```python
from build123d import *

# Parameters (mm, degrees)
SKETCH1_W           = 42
SKETCH1_H           = 42
SKETCH1_W_2         = 40
SKETCH1_H_2         = 40
BOSS_EXTRUDE1_DEPTH = 10
SKETCH3_W           = 2
SKETCH3_H           = 40
BOSS_EXTRUDE2_DEPTH = 40
SKETCH5_W           = 40
SKETCH5_H           = 1
CUT_EXTRUDE1_DEPTH  = 10
SKETCH6_W           = 40
SKETCH6_H           = 1
CUT_EXTRUDE2_DEPTH  = 10


with BuildPart() as part:
    # Sketch1 → Boss-Extrude1 (new body)
    with BuildSketch(Plane.XY):
        Rectangle(SKETCH1_W, SKETCH1_H)
        Rectangle(SKETCH1_W_2, SKETCH1_H_2, mode=Mode.SUBTRACT)
    extrude(amount=BOSS_EXTRUDE1_DEPTH)

    # Sketch3 → Boss-Extrude2 (add)
    with BuildSketch(Plane(origin=(-20, 0, 0), x_dir=(0, 0, -1), z_dir=(1, 0, 0))):
        with Locations((-1, 0)):
            Rectangle(SKETCH3_W, SKETCH3_H)
    extrude(amount=BOSS_EXTRUDE2_DEPTH)

    # Sketch5 → Cut-Extrude1 (cut)
    with BuildSketch(Plane.XY.offset(10)):
        with Locations((0, 20.5)):
            Rectangle(SKETCH5_W, SKETCH5_H)
    extrude(amount=-CUT_EXTRUDE1_DEPTH, mode=Mode.SUBTRACT)

    # Sketch6 → Cut-Extrude2 (cut)
    with BuildSketch(Plane.XY.offset(10)):
        with Locations((0, -20.5)):
            Rectangle(SKETCH6_W, SKETCH6_H)
    extrude(amount=-CUT_EXTRUDE2_DEPTH, mode=Mode.SUBTRACT)


solid = part.part
```
The model under review builds one solid part; all positions refer to its coordinate system, in mm. A direction names the side the tool comes from. Give positions to 0.01 mm unless a question says otherwise; leave off trailing zeros. Write each loop counter-clockwise with the first axis right and the second up, starting at its lowest first coordinate (ties: lowest second). Pieces come first, ordered by that corner, then holes. Notation, with made-up numbers: (-9, 58) - (8, 58) arc R23 cw to (8, 71) - close; hole circle Ø5 at (50, 76). An arc over 180 degrees is marked (long way). Answer in a Markdown table with one row per item. Add a question column.
1. Insertion check: P1, Ø3, axis at x = -14, y = 11, coming from the +Z side; P2, Ø1, axis at x = 7, z = 1, coming from the -Y side; P3, Ø2, axis at x = 6.5, z = 0.5, coming from the +Y side. Each pin has a flat end and moves straight along its axis. Give the tip position at first contact, or say it passes through.
2. We need section B-B on y = 12. Write out the cut boundary in (x, z), then the cut area to 3 significant figures.
3. Draft analysis for pull direction X (two halves, no side actions). For faces 4 (the flat face through (20.5, 21, 4.9)), 5 (the flat face through (-21, 0, 5)), 6 (the flat face through (0, -20, 1)), state which applies: +X half, -X half, draft (parallel to the pull), parting line (faces both ways), or undercut.
4. Tool access review of faces 1 (the flat face through (20.5, 0.3, 10)), 2 (the flat face through (0, 20, 1)), 3 (the flat face through (0, 0, 2)): name each direction out of +Z, -Z, +X, -X, +Y, -Y from which nothing blocks a thin tool from reaching the whole face with its end or side.
5. We need section A-A on z = 3. Write out the cut boundary in (x, y).
6. Wall thickness on line 1 along X through (y, z) = (-17, 2.75); line 2 along Z through (x, y) = (17.5, -16.5): over which ranges is each line inside the solid? List them lowest first. Write a range as [from, to].
7. We need section C-C on x = 6. Write out the cut boundary in (y, z), then the cut area to 3 significant figures.
Ans:
| question | item | result |
|---|---|---|
| 1 | P1 | stops at z = 2 |
| 1 | P2 | stops at y = -20 |
| 1 | P3 | stops at y = 20 |
| 2 | outline | (-21, 0) - (21, 0) - (21, 10) - (20, 10) - (20, 2) - (-20, 2) - (-20, 10) - (-21, 10) - close |
| 2 | area | 100 mm^2 |
| 3 | face 4 | draft |
| 3 | face 5 | -X half |
| 3 | face 6 | undercut |
| 4 | face 1 | +Z, +X, -X, +Y, -Y |
| 4 | face 2 | +Z, -Z, +Y |
| 4 | face 3 | +Z, +Y, -Y |
| 5 | outline | (-21, -21) - (-20, -21) - (-20, 21) - (-21, 21) - close; (20, -21) - (21, -21) - (21, 21) - (20, 21) - close |
| 6 | line 1 | x = [-21, -20], [20, 21] |
| 6 | line 2 | z = [0, 2] |
| 7 | outline | (-20, 0) - (20, 0) - (20, 2) - (-20, 2) - close |
| 7 | area | 80.0 mm^2 |
